Can you work these out from the drawing? Everything is in mm from the part's minimum corner. Coordinates: 2 decimals unless noted, no trailing zeros. Order: outer loops, then holes, each group sorted by start corner. A loop starts at its lowest first (then second) coordinate and runs counter-clockwise, first axis right, second up. Notation, with made-up numbers: (-30.5, 29.5) -> (-6.5, 29.5) arc R23 cw to (-6.5, 63.5) -> close; hole circle Ø7 at (29.5, -18.75). An arc over 180 degrees is marked (long way). Return JSON: item names as keys, results as strings. Group by question number.
1) For pin 1 (9 mm diameter, centred on x = 111.32, y = 51.36, fed in from +Z), with a flat end and sliding along its axis, tell me the tip position at first contact or that it passes through.
2) If I drill on probe 1 along X at (y, z) = (52, 80); probe 2 along Y at (x, z) = (18, 34) (1 decimal); probe 3 along X at (y, z) = (54, 15) (1 decimal), over which ranges is the centre line in solid material (lowest first)? Write a range as from..to.
3) If we section it at A-A, the plane z = 84.5: Please give me the cut outline in (x, y), then the cut area to 3 significant figures.
4) If we section it at B-B, the plane x = 109: Please give me the cut outline in (y, z) (1 decimal), then the cut area to 3 significant figures.
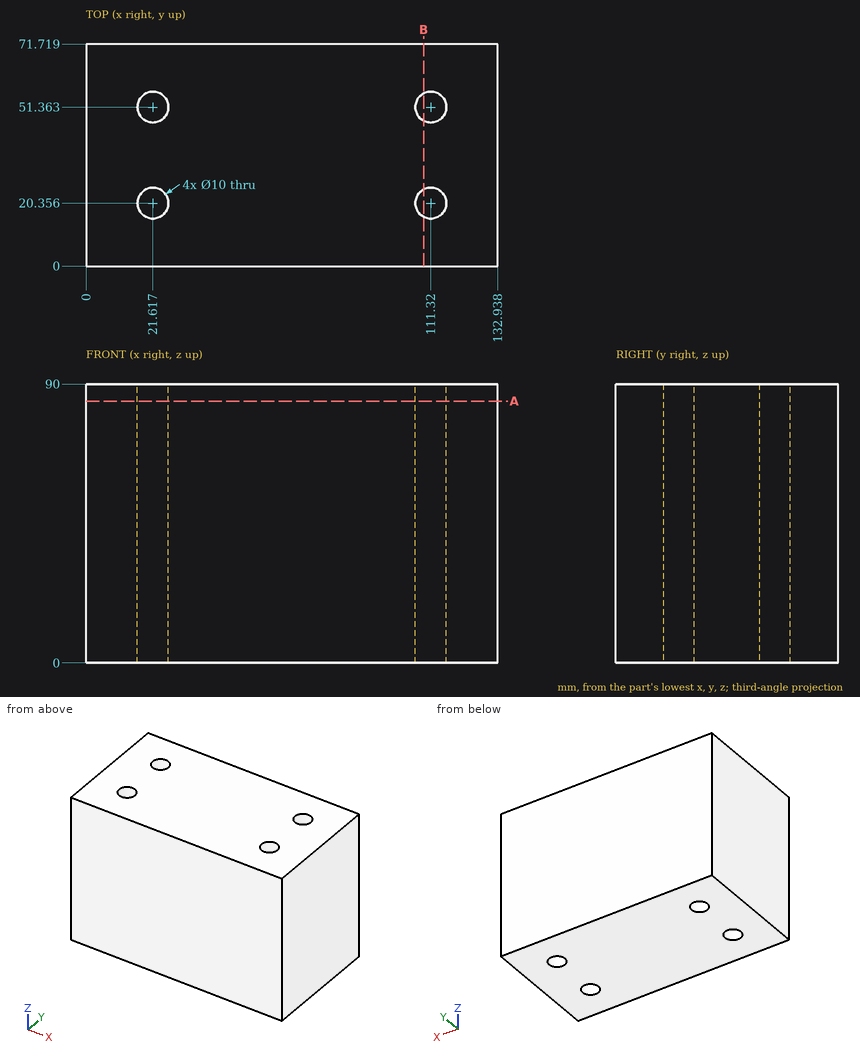
Result sheet:
{
 "1": {"pin 1": "passes through"},
 "2": {"probe 1": "x = 0..16.66, 26.58..106.36, 116.28..132.94", "probe 2": "y = 0..16.9, 23.8..47.9, 54.8..71.7", "probe 3": "x = 0..17.4, 25.9..107.1, 115.6..132.9"},
 "3": {"outline": "(0, 0) -> (132.94, 0) -> (132.94, 71.72) -> (0, 71.72) -> close; hole circle Ø10 at (21.62, 20.36); hole circle Ø10 at (21.62, 51.36); hole circle Ø10 at (111.32, 20.36); hole circle Ø10 at (111.32, 51.36)", "area": "9,220 mm2"},
 "4": {"outline": "(0, 0) -> (15.9, 0) -> (15.9, 90) -> (0, 90) -> close; (24.8, 0) -> (46.9, 0) -> (46.9, 90) -> (24.8, 90) -> close; (55.8, 0) -> (71.7, 0) -> (71.7, 90) -> (55.8, 90) -> close", "area": "4,860 mm2"}
}
